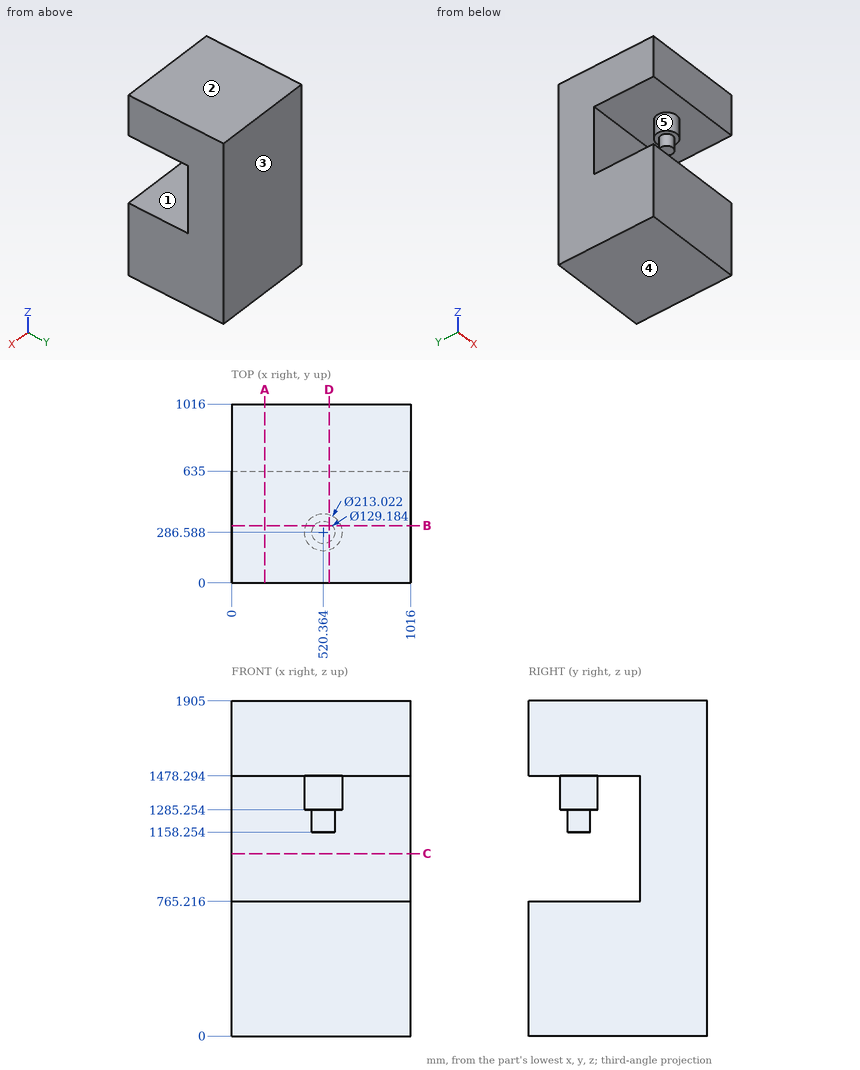
Verification items for this drawing (mm, ordinates from the low corner). A direction names the side the tool comes from. Coordinates: 2 decimals unless noted, no trailing zeros. Write each loop counter-clockwise with the first axis right and the second up, starting at its lowest first coordinate (ties: lowest second). Pieces come first, ordered by that corner, then holes. Notation, with made-up numbers: M 82.5,-9.75 L 137.5,-9.75 A12 cw 137.5,3.25 Z; hole C 28,74 d10. An arc over 180 degrees is marked long. One line per item, written item: value. Start each with the question number.
(1) Tool access check on the marked faces 1 and 2. Record the directions out of +Z, -Z, +X, -X, +Y, -Y that give a thin tool (end or side, any length) a straight path to the whole face; none if there is none.
(2) Sectioned sample at A-A, the plane x = 188.5. Enter the section's corners in (y, z), and give its area (3 significant figures).
(3) Sectioned sample at D-D, the plane x = 553. Enter the section's corners in (y, z) (1 decimal), and give its area (3 significant figures).
(4) Depth check by flat-ended pin: pin 1 (1 mm diameter, centred on x = 201, z = 1095, fed in from -Y); pin 2 (12 mm diameter, centred on x = 824.5, y = 347, fed in from -Z). Enter the tip coordinate at first touch or a pass-through.
(5) Scan lines: line 1 along Z through (x, y) = (840.5, 292); line 2 along Y through (x, z) = (292.5, 1018); line 3 along Y through (x, z) = (483, 1316.5) (1 decimal). Record each from-to range of solid material in increasing order. Write a range as [from, to].
(6) Sectioned sample at B-B, the plane y = 324.5. Enter the section's corners in (x, z), and give its area (3 significant figures).
(7) Sectioned sample at C-C, the plane z = 1036.5. Enter the section's corners in (x, y).
(8) Release check for a two-part mould opening along Z. For the marked faces 3, 4 and 5 record: released by +Z, released by -Z, zero draft, split by the parting line, or undercut.
Filled sheet:
1. face 1: +X, -X, -Y
1. face 2: +Z, +X, -X, +Y, -Y
2. outline: M 0,0 L 1016,0 L 1016,1905 L 0,1905 L 0,1478.29 L 635,1478.29 L 635,765.22 L 0,765.22 Z
2. area: 1,480,000 mm²
3. outline: M 0,0 L 1016,0 L 1016,1905 L 0,1905 L 0,1478.3 L 185.2,1478.3 L 185.2,1285.3 L 230.8,1285.3 L 230.8,1158.3 L 342.3,1158.3 L 342.3,1285.3 L 388,1285.3 L 388,1478.3 L 635,1478.3 L 635,765.2 L 0,765.2 Z
3. area: 1,540,000 mm²
4. pin 1: y = 635
4. pin 2: z = 0
5. line 1: [0, 765.22], [1478.29, 1905]
5. line 2: [635, 1016]
5. line 3: [186.8, 386.3], [635, 1016]
6. outline: M 0,0 L 1016,0 L 1016,765.22 L 0,765.22 Z; M 0,1478.29 L 420.83,1478.29 L 420.83,1285.25 L 468.07,1285.25 L 468.07,1158.25 L 572.66,1158.25 L 572.66,1285.25 L 619.9,1285.25 L 619.9,1478.29 L 1016,1478.29 L 1016,1905 L 0,1905 Z
6. area: 1,260,000 mm²
7. outline: M 0,635 L 1016,635 L 1016,1016 L 0,1016 Z
8. face 3: zero draft
8. face 4: released by -Z
8. face 5: undercut
